Read the model definition and answer for the solid it produces. Units are mm, in the model's axes. Face numbers are marked on the shaded views. A direction names the side the tool comes from. Coordinates: 2 decimals unless noted, no trailing zeros. Order: outer loops, then holes, each group sorted by start corner. A loop starts at its lowest first (then second) coordinate and runs counter-clockwise, first axis right, second up. Notation, with made-up numbers: (86, 69.25) -> (102, 69.25) arc R19 cw to (102, 104.25) -> close; hole circle Ø7 at (61.5, 11). An arc over 180 degrees is marked (long way). Answer as a JSON object with one key per item and string values. Group by question number.
1) Given pin 1 (2 mm diameter, centred on x = -5, y = 2.5, fed in from +Z); pin 2 (1.5 mm diameter, centred on y = 3.5, z = -10.5, fed in from -X); pin 3 (1 mm diameter, centred on x = -1.5, z = 4, fed in from +Y), each flat-ended and moving along its own axis, determine where each tip first touches the part or whether it passes through.
2) Section B-B on z = 1 is taken. Determine the outline of the cut face in (x, y), and give its area (3 significant figures).
3) Consider L1, parallel to Z at x = 0, y = -1.3 (3 decimals); L2, parallel to Y at x = 0, z = -14.15; L3, parallel to Z at x = -3.75, y = 2.75. Determine where each line is inside the solid, lowest interval first.
4) Section A-A on x = 0 is taken. Determine the outline of the cut face in (y, z) (3 decimals), and give its area (3 significant figures).
5) Section D-D on z = -9 is taken. Determine the outline of the cut face in (x, y) (3 decimals), and give its area (3 significant figures).
6) Determine the mould class of the marked faces 3, 4 and 5 for opening direction X: released by +X, released by -X, zero draft, split by the parting line, or undercut.
7) A tool of negligible diameter and unlimited length cuts with its end or side. For the marked faces 1 and 2, from which of +Z, -Z, +X, -X, +Y, -Y can it reach the whole face along a straight path? Write none if from no direction.
8) Section C-C on y = -2 is taken. Determine the outline of the cut face in (x, z) (3 decimals), and give its area (3 significant figures).
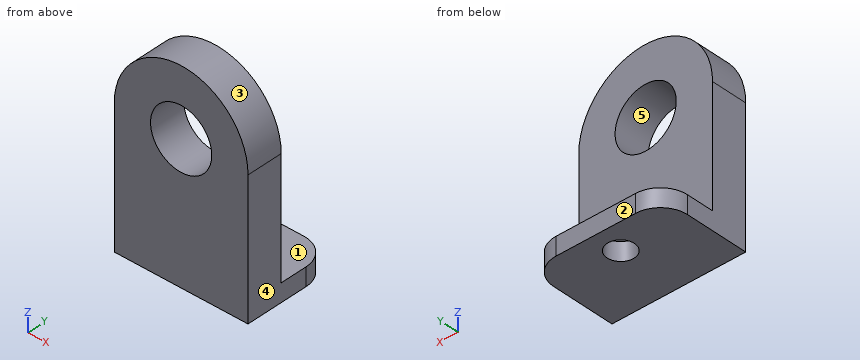
from build123d import *

# Parameters (mm, degrees)
F0_R     = 3.375
F1_DEPTH = 4
F2_W     = 14.75
F2_H     = 6
F2_H_2   = 4
F3_DEPTH = 2
F4_R     = 3
F5_D     = 3


# Not quite as in the source:
# - a feature names something its author has since deleted; it is built from what else it names


with BuildPart() as f1:
    # F0 (on Front) → F1 (new body)
    with BuildSketch(Plane.XZ):
        with BuildLine():
            Line((7.375, -15), (7.375, 0))
            ThreePointArc((7.375, 0), (0, -7.375), (-7.375, 0))
            Line((-7.375, 0), (-7.375, -15))
            Line((-7.375, -15), (7.375, -15))
        make_face()
        with BuildLine():
            ThreePointArc((-7.375, 0), (0, -7.375), (7.375, 0))
            ThreePointArc((7.375, 0), (0, 7.375), (-7.375, 0))
        make_face()
        Circle(F0_R, mode=Mode.SUBTRACT)
    extrude(amount=F1_DEPTH)

    # F2 (on face) → F3 (join)
    with BuildSketch(Plane(origin=(0, 0, -15), x_dir=(1, 0, 0), z_dir=(0, 0, -1))):
        with Locations((0, -3)):
            Rectangle(F2_W, F2_H)
        with Locations((0, 2)):
            Rectangle(F2_W, F2_H_2)
    extrude(amount=-F3_DEPTH)

    # F4
    f4_edges = [f1.edges().sort_by_distance(p)[0] for p in [
        (-7.375, 6, -14),
        (7.375, 6, -14),
    ]]
    fillet(f4_edges, radius=F4_R)

    # F5 (through all)
    with Locations(Plane(origin=(0, 0, -15), x_dir=(1, 0, 0), z_dir=(0, 0, -1))):
        with Locations((0, -3)):
            Hole(F5_D / 2)


solid = f1.part
Worked answers:
{
 "1": {"pin 1": "stops at z = -13", "pin 2": "passes through", "pin 3": "stops at y = 0"},
 "2": {"outline": "(-7.31, -4) -> (-3.22, -4) -> (-3.22, 0) -> (-7.31, 0) -> close; (3.22, -4) -> (7.31, -4) -> (7.31, 0) -> (3.22, 0) -> close", "area": "32.7 mm²"},
 "3": {"L1": "z = -15 to -3.375, 3.375 to 7.375", "L2": "y = -4 to 1.5, 4.5 to 6", "L3": "z = -15 to -13"},
 "4": {"outline": "(-4, -15) -> (1.5, -15) -> (1.5, -13) -> (0, -13) -> (0, -3.375) -> (-4, -3.375) -> close; (-4, 3.375) -> (0, 3.375) -> (0, 7.375) -> (-4, 7.375) -> close; (4.5, -15) -> (6, -15) -> (6, -13) -> (4.5, -13) -> close", "area": "68.5 mm²"},
 "5": {"outline": "(-7.375, -4) -> (7.375, -4) -> (7.375, 0) -> (-7.375, 0) -> close", "area": "59.0 mm²"},
 "6": {"face 3": "split by the parting line", "face 4": "released by +X", "face 5": "undercut"},
 "7": {"face 1": "+Z, +X, -X, +Y", "face 2": "+Z, -Z, +X, -X, +Y"},
 "8": {"outline": "(-7.375, -15) -> (7.375, -15) -> (7.375, 0) arc R7.375 ccw to (-7.375, 0) -> close; hole circle Ø6.75 at (0, 0)", "area": "271 mm²"}
}
